Answer from the drawing. Dimensions are ordinates in mm from the lowest x, y and z of the part. Give positions to 0.01 mm unless a question says otherwise; leave off trailing zeros. Order: outer loops, then holes, each group sorted by start corner. A loop starts at its lowest first (then second) coordinate and runs counter-clockwise, first axis right, second up.
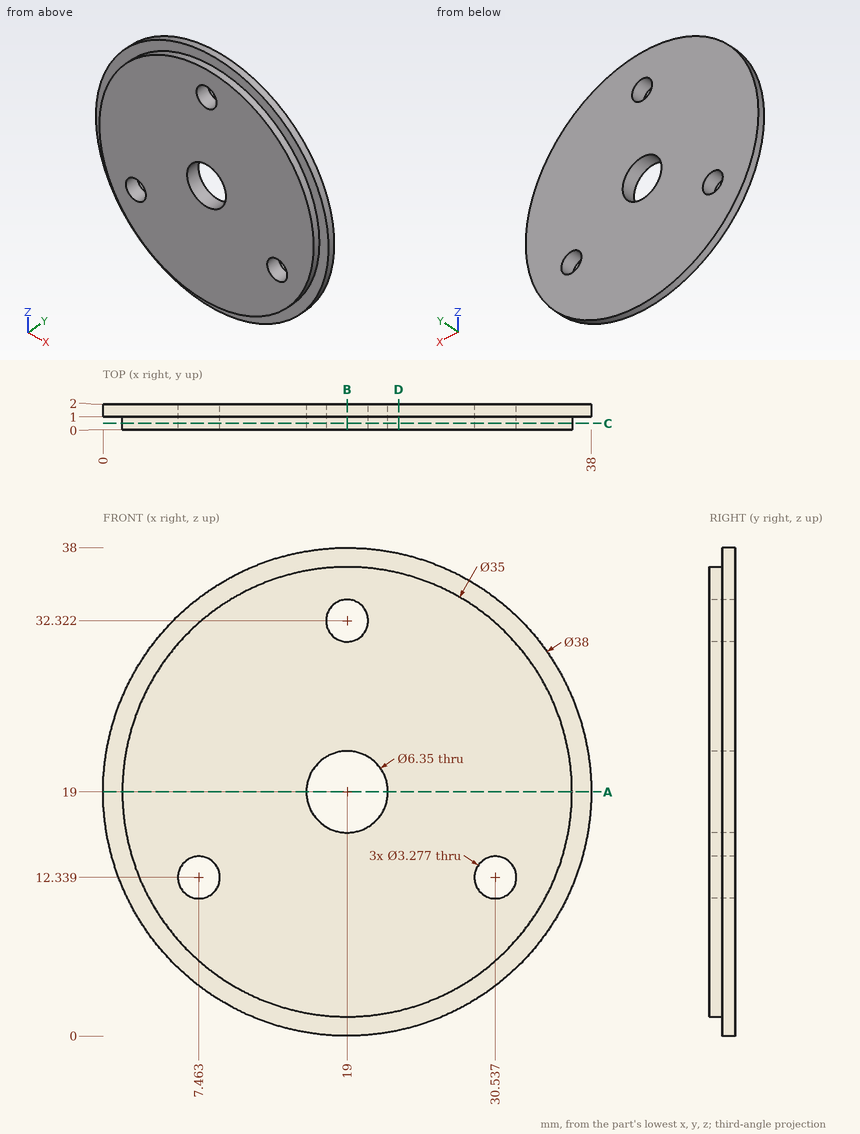
1) The part is cut by section C-C on y = 0.5. Count the separate pieces of the cut face and the enclosed holes in it, and give its area (3 significant figures).
Final values:
separate pieces: 1
enclosed holes: 4
area: 905 mm2
2) Given pin 1 (8 mm diameter, centred on x = 20.5, z = 7.5, fed in from -Y); pin 2 (2.5 mm diameter, centred on x = 7.46, z = 12.34, fed in from +Y), each flat-ended and moving along its own axis, determine where each tip first touches the part or whether it passes through.
Final values:
pin 1: stops at y = 0
pin 2: passes through
3) Consider L1, parallel to Z at x = 19, y = 1.5 (1 decimal); L2, parallel to Z at x = 19, y = 0.75 (1 decimal); L3, parallel to Y at x = 36.5, z = 22.5. Determine where each line is inside the solid, lowest interval first.
Final values:
L1: z = 0 to 15.8, 22.2 to 30.7, 34 to 38
L2: z = 1.5 to 15.8, 22.2 to 30.7, 34 to 36.5
L3: y = 1 to 2
4) The part is cut by section B-B on x = 19. Determine the outline of the cut face in (y, z) (1 decimal).
Final values:
outline: (0, 1.5) - (1, 1.5) - (1, 0) - (2, 0) - (2, 15.8) - (0, 15.8) - close; (0, 22.2) - (2, 22.2) - (2, 30.7) - (0, 30.7) - close; (0, 34) - (2, 34) - (2, 38) - (1, 38) - (1, 36.5) - (0, 36.5) - close
5) The part is cut by section D-D on x = 23. Determine the outline of the cut face in (y, z).
Final values:
outline: (0, 1.96) - (1, 1.96) - (1, 0.43) - (2, 0.43) - (2, 37.57) - (1, 37.57) - (1, 36.04) - (0, 36.04) - close
6) The part is cut by section A-A on z = 19. Determine the outline of the cut face in (x, y) (1 decimal).
Final values:
outline: (0, 1) - (1.5, 1) - (1.5, 0) - (15.8, 0) - (15.8, 2) - (0, 2) - close; (22.2, 0) - (36.5, 0) - (36.5, 1) - (38, 1) - (38, 2) - (22.2, 2) - close
